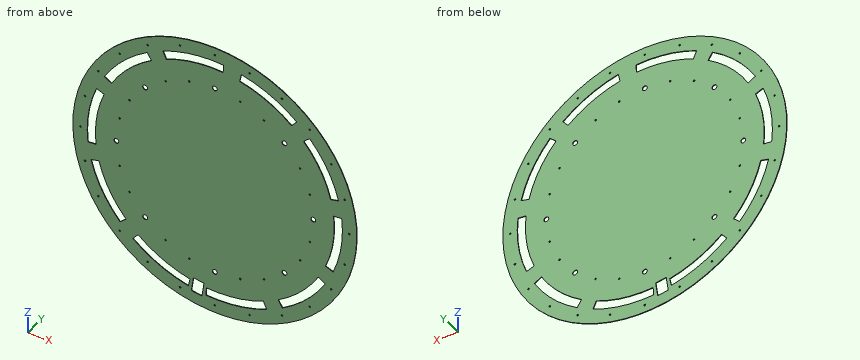
```python
from build123d import *

# Parameters (mm, degrees)
SKETCH1_R           = 346
SKETCH1_R_2         = 6
SKETCH1_R_3         = 2
BOSS_EXTRUDE1_DEPTH = 0.75


with BuildPart() as part:
    # Sketch1 → Boss-Extrude1 (new, symmetric)
    with BuildSketch(Plane(origin=(0, 0, 0), x_dir=(1, 0, 0), z_dir=(0, 1, 0))):
        with Locations(Location((0, 0, 0), (0, 0, 270))):
            Circle(SKETCH1_R)
        with Locations(Location((0, 240, 0), (0, 0, 270))):
            Circle(SKETCH1_R_2, mode=Mode.SUBTRACT)
        with Locations(Location((169.705627485, 169.705627485, 0), (0, 0, 270))):
            Circle(SKETCH1_R_2, mode=Mode.SUBTRACT)
        with Locations(Location((240, 0, 0), (0, 0, 270))):
            Circle(SKETCH1_R_2, mode=Mode.SUBTRACT)
        with Locations(Location((169.705627485, -169.705627485, 0), (0, 0, 270))):
            Circle(SKETCH1_R_2, mode=Mode.SUBTRACT)
        with Locations(Location((0, -240, 0), (0, 0, 270))):
            Circle(SKETCH1_R_2, mode=Mode.SUBTRACT)
        with Locations(Location((-169.705627485, -169.705627485, 0), (0, 0, 270))):
            Circle(SKETCH1_R_2, mode=Mode.SUBTRACT)
        with Locations(Location((-240, 0, 0), (0, 0, 270))):
            Circle(SKETCH1_R_2, mode=Mode.SUBTRACT)
        with Locations(Location((-169.705627485, 169.705627485, 0), (0, 0, 270))):
            Circle(SKETCH1_R_2, mode=Mode.SUBTRACT)
        with Locations(Location((-231.822198309, 62.116570825, 0), (0, 0, 270))):
            Circle(SKETCH1_R_3, mode=Mode.SUBTRACT)
        with Locations(Location((-207.846062834, 120.000258819, 0), (0, 0, 270))):
            Circle(SKETCH1_R_3, mode=Mode.SUBTRACT)
        with Locations(Location((-119.999707107, 207.846804015, 0), (0, 0, 270))):
            Circle(SKETCH1_R_3, mode=Mode.SUBTRACT)
        with Locations(Location((-62.116070825, 231.823064335, 0), (0, 0, 270))):
            Circle(SKETCH1_R_3, mode=Mode.SUBTRACT)
        with Locations(Location((62.117570825, 231.823198309, 0), (0, 0, 270))):
            Circle(SKETCH1_R_3, mode=Mode.SUBTRACT)
        with Locations(Location((120.001258819, 207.847062834, 0), (0, 0, 270))):
            Circle(SKETCH1_R_3, mode=Mode.SUBTRACT)
        with Locations(Location((207.847804015, 120.000707107, 0), (0, 0, 270))):
            Circle(SKETCH1_R_3, mode=Mode.SUBTRACT)
        with Locations(Location((231.824064335, 62.117070825, 0), (0, 0, 270))):
            Circle(SKETCH1_R_3, mode=Mode.SUBTRACT)
        with Locations(Location((231.824198309, -62.116570825, 0), (0, 0, 270))):
            Circle(SKETCH1_R_3, mode=Mode.SUBTRACT)
        with Locations(Location((207.848062834, -120.000258819, 0), (0, 0, 270))):
            Circle(SKETCH1_R_3, mode=Mode.SUBTRACT)
        with Locations(Location((120.001707107, -207.846804015, 0), (0, 0, 270))):
            Circle(SKETCH1_R_3, mode=Mode.SUBTRACT)
        with Locations(Location((62.118070825, -231.823064335, 0), (0, 0, 270))):
            Circle(SKETCH1_R_3, mode=Mode.SUBTRACT)
        with Locations(Location((-62.115570825, -231.823198309, 0), (0, 0, 270))):
            Circle(SKETCH1_R_3, mode=Mode.SUBTRACT)
        with Locations(Location((-119.999258819, -207.847062834, 0), (0, 0, 270))):
            Circle(SKETCH1_R_3, mode=Mode.SUBTRACT)
        with Locations(Location((-207.845804015, -120.000707107, 0), (0, 0, 270))):
            Circle(SKETCH1_R_3, mode=Mode.SUBTRACT)
        with Locations(Location((-231.822064335, -62.117070825, 0), (0, 0, 270))):
            Circle(SKETCH1_R_3, mode=Mode.SUBTRACT)
        with Locations(Location((-316.34070811, 84.763237271, 0), (0, 0, 270))):
            Circle(SKETCH1_R_3, mode=Mode.SUBTRACT)
        with Locations(Location((-283.623319739, 163.75, 0), (0, 0, 270))):
            Circle(SKETCH1_R_3, mode=Mode.SUBTRACT)
        with Locations(Location((-231.577470839, 231.577470839, 0), (0, 0, 270))):
            Circle(SKETCH1_R_3, mode=Mode.SUBTRACT)
        with Locations(Location((-163.75, 283.623319739, 0), (0, 0, 270))):
            Circle(SKETCH1_R_3, mode=Mode.SUBTRACT)
        with Locations(Location((-84.763237271, 316.34070811, 0), (0, 0, 270))):
            Circle(SKETCH1_R_3, mode=Mode.SUBTRACT)
        with Locations(Location((0, 327.5, 0), (0, 0, 270))):
            Circle(SKETCH1_R_3, mode=Mode.SUBTRACT)
        with Locations(Location((84.763237271, 316.34070811, 0), (0, 0, 270))):
            Circle(SKETCH1_R_3, mode=Mode.SUBTRACT)
        with Locations(Location((163.75, 283.623319739, 0), (0, 0, 270))):
            Circle(SKETCH1_R_3, mode=Mode.SUBTRACT)
        with Locations(Location((231.577470839, 231.577470839, 0), (0, 0, 270))):
            Circle(SKETCH1_R_3, mode=Mode.SUBTRACT)
        with Locations(Location((283.623319739, 163.75, 0), (0, 0, 270))):
            Circle(SKETCH1_R_3, mode=Mode.SUBTRACT)
        with Locations(Location((316.34070811, 84.763237271, 0), (0, 0, 270))):
            Circle(SKETCH1_R_3, mode=Mode.SUBTRACT)
        with Locations(Location((327.5, 0, 0), (0, 0, 270))):
            Circle(SKETCH1_R_3, mode=Mode.SUBTRACT)
        with Locations(Location((316.34070811, -84.763237271, 0), (0, 0, 270))):
            Circle(SKETCH1_R_3, mode=Mode.SUBTRACT)
        with Locations(Location((283.623319739, -163.75, 0), (0, 0, 270))):
            Circle(SKETCH1_R_3, mode=Mode.SUBTRACT)
        with Locations(Location((231.577470839, -231.577470839, 0), (0, 0, 270))):
            Circle(SKETCH1_R_3, mode=Mode.SUBTRACT)
        with Locations(Location((163.75, -283.623319739, 0), (0, 0, 270))):
            Circle(SKETCH1_R_3, mode=Mode.SUBTRACT)
        with Locations(Location((84.763237271, -316.34070811, 0), (0, 0, 270))):
            Circle(SKETCH1_R_3, mode=Mode.SUBTRACT)
        with Locations(Location((0, -327.5, 0), (0, 0, 270))):
            Circle(SKETCH1_R_3, mode=Mode.SUBTRACT)
        with Locations(Location((-84.763237271, -316.34070811, 0), (0, 0, 270))):
            Circle(SKETCH1_R_3, mode=Mode.SUBTRACT)
        with Locations(Location((-163.75, -283.623319739, 0), (0, 0, 270))):
            Circle(SKETCH1_R_3, mode=Mode.SUBTRACT)
        with Locations(Location((-231.577470839, -231.577470839, 0), (0, 0, 270))):
            Circle(SKETCH1_R_3, mode=Mode.SUBTRACT)
        with Locations(Location((-283.623319739, -163.75, 0), (0, 0, 270))):
            Circle(SKETCH1_R_3, mode=Mode.SUBTRACT)
        with Locations(Location((-316.34070811, -84.763237271, 0), (0, 0, 270))):
            Circle(SKETCH1_R_3, mode=Mode.SUBTRACT)
        with Locations(Location((-327.5, 0, 0), (0, 0, 270))):
            Circle(SKETCH1_R_3, mode=Mode.SUBTRACT)
        Polygon((-57.130530999, 313.095995547), (-31.383561212, 316.714496172), (-26.373329577, 281.064845698), (-52.120299364, 277.446345073), align=None, mode=Mode.SUBTRACT)
        with BuildLine():
            Line((-20.29913386, 290.291138626), (-21.694263334, 310.242419631))
            ThreePointArc((-21.694263334, 310.242419631), (54.004583254, 306.275211187), (126.495095997, 284.112637327))
            Line((126.495095997, 284.112637327), (118.360363135, 265.841728174))
            ThreePointArc((118.360363135, 265.841728174), (50.531619701, 286.579056127), (-20.29913386, 290.291138626))
        make_face(mode=Mode.SUBTRACT)
        with BuildLine():
            Line((269.333900577, 155.5), (252.013392501, 145.5))
            ThreePointArc((252.013392501, 145.5), (209.327881899, 202.145585804), (154.206505892, 246.781995982))
            Line((154.206505892, 246.781995982), (164.804891177, 263.742957905))
            ThreePointArc((164.804891177, 263.742957905), (223.714677905, 216.038753213), (269.333900577, 155.5))
        make_face(mode=Mode.SUBTRACT)
        with BuildLine():
            Line((309.29630946, -32.508352076), (289.405871552, -30.417782811))
            ThreePointArc((289.405871552, -30.417782811), (288.168008004, 40.499372379), (269.810501679, 109.010518684))
            Line((269.810501679, 109.010518684), (288.35417877, 116.502650552))
            ThreePointArc((288.35417877, 116.502650552), (307.973369379, 43.282834399), (309.29630946, -32.508352076))
        make_face(mode=Mode.SUBTRACT)
        with BuildLine():
            Line((231.118040723, -208.099618578), (216.255144214, -194.71700645))
            ThreePointArc((216.255144214, -194.71700645), (256.937749522, -136.616224771), (282.356056346, -70.39927162))
            Line((282.356056346, -70.39927162), (301.761970872, -75.237709532))
            ThreePointArc((301.761970872, -75.237709532), (274.596701379, -146.005656026), (231.118040723, -208.099618578))
        make_face(mode=Mode.SUBTRACT)
        with BuildLine():
            Line((64.660535844, -304.203903828), (60.502302028, -284.640951814))
            ThreePointArc((60.502302028, -284.640951814), (127.566003716, -261.549067473), (187.051194419, -222.918932948))
            Line((187.051194419, -222.918932948), (199.906946613, -238.23982181))
            ThreePointArc((199.906946613, -238.23982181), (136.333426651, -279.524948399), (64.660535844, -304.203903828))
        make_face(mode=Mode.SUBTRACT)
        with BuildLine():
            Line((-126.495095997, -284.112637327), (-118.360363135, -265.841728174))
            ThreePointArc((-118.360363135, -265.841728174), (-50.531619701, -286.579056127), (20.29913386, -290.291138626))
            Line((20.29913386, -290.291138626), (21.694263334, -310.242419631))
            ThreePointArc((21.694263334, -310.242419631), (-54.004583254, -306.275211187), (-126.495095997, -284.112637327))
        make_face(mode=Mode.SUBTRACT)
        with BuildLine():
            Line((-269.333900577, -155.5), (-252.013392501, -145.5))
            ThreePointArc((-252.013392501, -145.5), (-209.327881899, -202.145585804), (-154.206505892, -246.781995982))
            Line((-154.206505892, -246.781995982), (-164.804891177, -263.742957905))
            ThreePointArc((-164.804891177, -263.742957905), (-223.714677905, -216.038753213), (-269.333900577, -155.5))
        make_face(mode=Mode.SUBTRACT)
        with BuildLine():
            Line((-309.29630946, 32.508352076), (-289.405871552, 30.417782811))
            ThreePointArc((-289.405871552, 30.417782811), (-288.168008004, -40.499372379), (-269.810501679, -109.010518684))
            Line((-269.810501679, -109.010518684), (-288.35417877, -116.502650552))
            ThreePointArc((-288.35417877, -116.502650552), (-307.973369379, -43.282834399), (-309.29630946, 32.508352076))
        make_face(mode=Mode.SUBTRACT)
        with BuildLine():
            Line((-231.118040723, 208.099618578), (-216.255144214, 194.71700645))
            ThreePointArc((-216.255144214, 194.71700645), (-256.937749522, 136.616224771), (-282.356056346, 70.39927162))
            Line((-282.356056346, 70.39927162), (-301.761970872, 75.237709531))
            ThreePointArc((-301.761970872, 75.237709531), (-274.596701379, 146.005656026), (-231.118040723, 208.099618578))
        make_face(mode=Mode.SUBTRACT)
        with BuildLine():
            Line((-64.660535844, 304.203903828), (-60.502302028, 284.640951814))
            ThreePointArc((-60.502302028, 284.640951814), (-127.566003716, 261.549067473), (-187.051194419, 222.918932948))
            Line((-187.051194419, 222.918932948), (-199.906946612, 238.23982181))
            ThreePointArc((-199.906946612, 238.23982181), (-136.333426651, 279.524948399), (-64.660535844, 304.203903828))
        make_face(mode=Mode.SUBTRACT)
    extrude(amount=BOSS_EXTRUDE1_DEPTH, both=True)


solid = part.part
```
Work out the finished part from the listing and answer in its coordinate system (mm). Give positions to 0.01 mm unless a question says otherwise; leave off trailing zeros.
1. Section A-A, the plane y = -0.3 is taken. Give the number of separate pieces and of enclosed holes in the cut face, and give its area (3 significant figures).
Result sheet:
separate pieces: 1
enclosed holes: 59
area: 344,000 mm2
2. Each of these flat-tipped pins is pushed along its axis until it touches: P1, Ø2.5, axis at x = 231.58, z = 231.58, coming from the -Y side (3 decimals); P2, Ø6.5, axis at x = 327.5, z = 0, coming from the -Y side. Where does it stop, or does it pass through?
Result sheet:
P1: passes through
P2: stops at y = -0.75
3. Straight lines are drawn through the part: L1, parallel to Z at x = 9, y = -0.1; L2, parallel to Z at x = -73.5, y = 0.7; L3, parallel to X at y = -0.45, z = 197. For each, find the intervals that lie inside material, in ascending order.
Result sheet:
L1: z = -345.88 to -310.87, -290.86 to 290.86, 310.87 to 345.88
L2: z = -338.1 to -302.19, -281.56 to 281.56, 302.19 to 338.1
L3: x = -284.44 to -240.65, -214.18 to 218.79, 240.65 to 284.44
